Autodesk Inventor part; units mm, degrees
ref_plane "YZ Plane" through (0, 0, 0) normal (1, 0, 0) x (0, 1, 0)
ref_plane "XZ Plane" through (0, 0, 0) normal (0, 1, 0) x (-1, 0, 0)
ref_plane "XY Plane" through (0, 0, 0) normal (0, 0, 1) x (1, 0, 0)
sketch "스케치1" plane through (0, 0, 0) normal (0, 1, 0) x (-1, 0, 0)
  line L0 (-68, 40) -> (68, 40)
  line L1 (68, 40) -> (68, -40)
  line L2 (68, -40) -> (-68, -40)
  line L3 (-68, -40) -> (-68, 40)
  line L4 (-68, 40) -> (68, -40) construction
  line L5 (68, 40) -> (-68, -40) construction
  point P0 (0, 0)
  dimension "d0" = 136
  dimension "d1" = 80
extrude "돌출1" add sketch "스케치1" along normal blind 3
sketch "스케치2" plane through (0, 3, 0) normal (0, 1, 0) x (1, 0, 0)
  circle A0 centre (-54.5, 24.5) radius 1.75
  circle A1 centre (-5.5, 24.5) radius 1.75
  circle A2 centre (5.5, 24.5) radius 1.75
  circle A3 centre (54.5, 24.5) radius 1.75
  circle A4 centre (54.5, -24.5) radius 1.75
  circle A5 centre (5.5, -24.5) radius 1.75
  circle A6 centre (-5.5, -24.5) radius 1.75
  circle A7 centre (-54.5, -24.5) radius 1.75
  circle A8 centre (-61, 36) radius 2
  line L0 (-65, 32) -> (-57, 32)
  line L1 (-57, 32) -> (-57, 40)
  line L2 (-57, 40) -> (-65, 40)
  line L3 (-65, 40) -> (-65, 32)
  line L4 (-65, 32) -> (-57, 40) construction
  line L5 (-57, 32) -> (-65, 40) construction
  line L6 (68, 40) -> (-68, 40)
  line L7 (-68, 40) -> (-68, -40)
  line L8 (-1.8724, 0) -> (2.8404, 0)
  line L9 (0, 1.8083) -> (0, -2.4649)
  circle A9 centre (61, 36) radius 2
  circle A10 centre (-61, -36) radius 2
  circle A11 centre (61, -36) radius 2
  line L10 (68, -40) -> (68, 40)
  line L11 (-68, -40) -> (68, -40)
  dimension "d13" = 3.5
  dimension "d14" = 3.5
  dimension "d15" = 3.5
  dimension "d16" = 3.5
  dimension "d17" = 3.5
  dimension "d18" = 3.5
  dimension "d19" = 3.5
  dimension "d20" = 3.5
  dimension "d21" = 4
  dimension "d22" = 8
  dimension "d23" = 4
  dimension "d24" = 8
  dimension "d25" = 7
  dimension "d26" = 13.5
  dimension "d27" = 13.5
  dimension "d28" = 13.5
  dimension "d29" = 13.5
  dimension "d30" = 0
  dimension "d31" = 0
  dimension "d32" = 0
  dimension "d33" = 0
  dimension "d34" = 0
  dimension "d35" = 0
  dimension "d36" = 0
  dimension "d37" = 0
  dimension "d38" = 49
  dimension "d39" = 11
  dimension "d40" = 49
  dimension "d41" = 15.5
extrude "돌출2" cut sketch "스케치2" against normal blind 3 contours A0 | A1 | A2 | A3 | A4 | A5 | A6 | A7 | A8 | A9 | A10 | A11
equation "\"d27\" = d26"
equation "\"d28\" = d26"
equation "\"d29\" = d26"
properties part number "라즈베리파이 보관소 2층 판"
The listing builds one solid part. Answer for the finished solid, in the listing's coordinates (mm). Coordinates: 2 decimals unless noted, no trailing zeros. Loops run counter-clockwise (first coordinate to the right, second up) from the corner with the lowest first, then second, coordinate; pieces in that order, holes last. Notation, with made-up numbers: (3.5, 13.5) -> (12.5, 13.5) arc R15 cw to (12.5, 35.5) -> close; hole circle Ø11 at (-2, 18). An arc over 180 degrees is marked (long way). Write item = value, one per line. Start each with the question number.
1) Given pin 1 Ø5.5 at (x, z) = (5.5, 24.5) entering from -Y; pin 2 Ø3 at (x, z) = (54.5, -24.5) entering from +Y, each flat-ended and moving along its own axis, determine where each tip first touches the part or whether it passes through.
2) A cutting plane is placed at A-A (x = 5.5). Give the vertices of the cut face in (y, z), then the cut area to 3 significant figures.
3) A cutting plane is placed at C-C (z = 24.5). Give the vertices of the cut face in (x, y).
4) A cutting plane is placed at B-B (z = 36). Give the vertices of the cut face in (x, y).
5) Straight lines are drawn through the part: line 1 (Z direction, x = 5.5, y = 1.95); line 2 (Z direction, x = -61, y = 0.9); line 3 (X direction, y = 2.15, z = 25). For each, find the intervals that lie inside material, in ascending order. Write a range as from..to.
6) The mould has two halves that part along X. Classify faces 1 (the face through (1, 1, 40)), 2 (the face through (-61, 2, -34)), 3 (the face through (68, 1, -1)): released by +X, released by -X, zero draft, split by the parting line, or undercut.
Responses:
q1.pin_1 = 0
q1.pin_2 = through
q2.outline = (0, -40) -> (3, -40) -> (3, -26.25) -> (0, -26.25) -> close; (0, -22.75) -> (3, -22.75) -> (3, 22.75) -> (0, 22.75) -> close; (0, 26.25) -> (3, 26.25) -> (3, 40) -> (0, 40) -> close
q2.area = 219 mm²
q3.outline = (-68, 0) -> (-56.25, 0) -> (-56.25, 3) -> (-68, 3) -> close; (-52.75, 0) -> (-7.25, 0) -> (-7.25, 3) -> (-52.75, 3) -> close; (-3.75, 0) -> (3.75, 0) -> (3.75, 3) -> (-3.75, 3) -> close; (7.25, 0) -> (52.75, 0) -> (52.75, 3) -> (7.25, 3) -> close; (56.25, 0) -> (68, 0) -> (68, 3) -> (56.25, 3) -> close
q4.outline = (-68, 0) -> (-63, 0) -> (-63, 3) -> (-68, 3) -> close; (-59, 0) -> (59, 0) -> (59, 3) -> (-59, 3) -> close; (63, 0) -> (68, 0) -> (68, 3) -> (63, 3) -> close
q5.line_1 = -40..-26.25, -22.75..22.75, 26.25..40
q5.line_2 = -40..-38, -34..34, 38..40
q5.line_3 = -68..-56.18, -52.82..-7.18, -3.82..3.82, 7.18..52.82, 56.18..68
q6.face_1 = zero draft
q6.face_2 = undercut
q6.face_3 = released by +X
